Autodesk Inventor part; units mm, degrees
ref_plane "YZ Plane" through (0, 0, 0) normal (1, 0, 0) x (0, 1, 0)
ref_plane "XZ Plane" through (0, 0, 0) normal (0, 1, 0) x (-1, 0, 0)
ref_plane "XY Plane" through (0, 0, 0) normal (0, 0, 1) x (1, 0, 0)
sketch "Sketch1" plane through (0, 0, 0) normal (1, 0, 0) x (0, 1, 0)
  circle A0 centre (0, 0) radius 11.5
  line L0 (0, 0) -> (0, -12.7) construction
  line L1 (0, -12.7) -> (6.35, -12.7) construction
  circle A1 centre (6.35, -12.7) radius 1.7526
  circle A2 centre (-6.35, -12.7) radius 1.7526
  circle A3 centre (6.35, 12.7) radius 1.7526
  circle A4 centre (-6.35, 12.7) radius 1.7526
  line L2 (12.7, 15.875) -> (-12.7, 15.875)
  line L3 (-12.7, 15.875) -> (-12.7, -15.875)
  line L4 (-12.7, -15.875) -> (12.7, -15.875)
  line L5 (12.7, -15.875) -> (12.7, 15.875)
  line L6 (12.7, 15.875) -> (-12.7, -15.875) construction
  line L7 (-12.7, 15.875) -> (12.7, -15.875) construction
  line L8 (0, 0) -> (9, 0) construction
  dimension "d0" = 23
  dimension "d1" = 12.7
  dimension "d2" = 6.35
  dimension "d3" = 3.5052
  dimension "d6" = 12.7
  dimension "d9" = 25.4
  dimension "d12" = 25.4
  dimension "d13" = 31.75
  dimension "d15" = 9
extrude "Extrusion1" add sketch "Sketch1" along normal blind 3.175
fillet "Fillet1" radius 3.175 4 edges at (1.5875, 12.7, 15.875) (1.5875, -12.7, 15.875) (1.5875, 12.7, -15.875) (1.5875, -12.7, -15.875)
equation "\"d9\" = 2 * d1"
properties part number "Motor Plates" material "UHMW, Black"
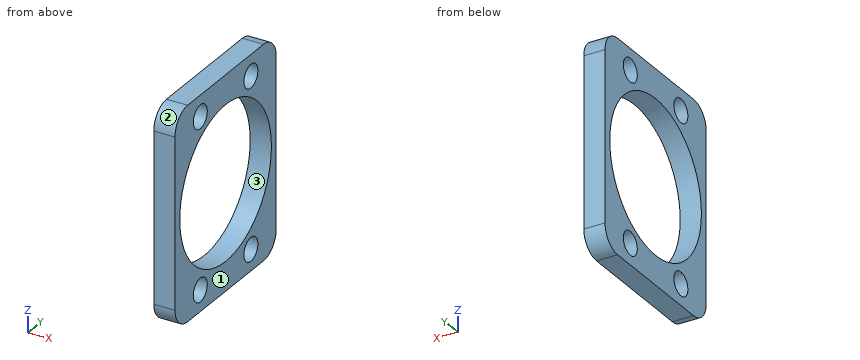
Here's how the part is built. I have some questions about the finished solid (model axes, mm). Face numbers are marked on the shaded views. Coordinates: 2 decimals unless noted, no trailing zeros. Order: outer loops, then holes, each group sorted by start corner. A loop starts at its lowest first (then second) coordinate and runs counter-clockwise, first axis right, second up. Notation, with made-up numbers: M -12,35 L 47,35 A26 ccw 47,69 Z; hole C 36.5,-28 d6. An arc over 180 degrees is marked long. Answer as a JSON object with one key per item and string values. Group by question number.
(1) I need wall thicknesses on probe 1 along Z at (x, y) = (2.05, -3.5) (3 decimals); probe 2 along Z at (x, y) = (1.35, 6.35) (3 decimals); probe 3 along Z at (x, y) = (0.95, -5) (3 decimals). Which ranges of each line are inside material? Lowest first, please.
(2) Suppose I cut it at A-A, the plane y = 0. Please give me the cut outline in (x, z) (3 decimals), then the cut area to 3 significant figures.
(3) Suppose I cut it at C-C, the plane z = -2.5. Please give me the cut outline in (x, y) (3 decimals).
(4) Suppose I cut it at D-D, the plane y = -6.75. Please give me the cut outline in (x, z) (3 decimals), then the cut area to 3 significant figures.
(5) For pin 1 (14 mm diameter, centred on y = 0, z = 0, fed in from -X), with a flat end and sliding along its axis, tell me the tip position at first contact or that it passes through.
(6) Suppose I cut it at B-B, the plane x = 0.5. Please give me the cut outline in (y, z) (3 decimals).
(7) If we mould it in two halves opening along Y, with no side actions, what happens to the marked faces 1, 2 and 3? For each: released by +Y, released by -Y, zero draft, split by the parting line, or undercut.
Values found:
{
 "1": {"probe 1": "z = -15.875 to -10.954, 10.954 to 15.875", "probe 2": "z = -15.875 to -14.453, -10.947 to -9.588, 9.588 to 10.947, 14.453 to 15.875", "probe 3": "z = -15.875 to -13.818, -11.582 to -10.356, 10.356 to 11.582, 13.818 to 15.875"},
 "2": {"outline": "M 0,-15.875 L 3.175,-15.875 L 3.175,-11.5 L 0,-11.5 Z; M 0,11.5 L 3.175,11.5 L 3.175,15.875 L 0,15.875 Z", "area": "27.8 mm^2"},
 "3": {"outline": "M 0,-12.7 L 3.175,-12.7 L 3.175,-11.225 L 0,-11.225 Z; M 0,11.225 L 3.175,11.225 L 3.175,12.7 L 0,12.7 Z"},
 "4": {"outline": "M 0,-15.875 L 3.175,-15.875 L 3.175,-14.406 L 0,-14.406 Z; M 0,-10.994 L 3.175,-10.994 L 3.175,-9.311 L 0,-9.311 Z; M 0,9.311 L 3.175,9.311 L 3.175,10.994 L 0,10.994 Z; M 0,14.406 L 3.175,14.406 L 3.175,15.875 L 0,15.875 Z", "area": "20.0 mm^2"},
 "5": {"pin 1": "passes through"},
 "6": {"outline": "M -12.7,-12.7 A3.175 ccw -9.525,-15.875 L 9.525,-15.875 A3.175 ccw 12.7,-12.7 L 12.7,12.7 A3.175 ccw 9.525,15.875 L -9.525,15.875 A3.175 ccw -12.7,12.7 Z; hole C 0,0 d23; hole C -6.35,-12.7 d3.505; hole C -6.35,12.7 d3.505; hole C 6.35,-12.7 d3.505; hole C 6.35,12.7 d3.505"},
 "7": {"face 1": "zero draft", "face 2": "released by -Y", "face 3": "undercut"}
}
